```python
from build123d import *

# Parameters (mm, degrees)
BOSS_EXTRUDE1_DEPTH          = 40
SKETCH2_W                    = 3.5
SKETCH2_H                    = 40
BOSS_EXTRUDE2_DEPTH          = 5
SKETCH4_R                    = 2
CUT_EXTRUDE1_DEPTH           = 7
SKETCH5_R                    = 3.5
CUT_EXTRUDE2_DEPTH           = 3
CUT_EXTRUDE2_DRAFT           = -27
CUT_EXTRUDE2_PROFILE_2_DEPTH = 3
CUT_EXTRUDE2_PROFILE_2_DRAFT = -27
BOSS_EXTRUDE3_DEPTH          = 3
SKETCH9_W                    = 13
SKETCH9_H                    = 40
CUT_EXTRUDE4_DEPTH           = 4.702585656
SKETCH10_W                   = 15
SKETCH10_H                   = 40
BOSS_EXTRUDE4_DEPTH          = 2.5
SKETCH11_W                   = 1.5
SKETCH11_H                   = 2.202585656
BOSS_EXTRUDE7_DEPTH          = 40
BOSS_EXTRUDE8_DEPTH          = 0.625841469
SKETCH13_R                   = 2
CUT_EXTRUDE5_DEPTH           = 10
SKETCH14_W                   = 2.5
SKETCH14_H                   = 40
BOSS_EXTRUDE9_DEPTH          = 0.5
SKETCH15_W                   = 2.5
SKETCH15_H                   = 40
BOSS_EXTRUDE10_DEPTH         = 0.5
BOSS_EXTRUDE11_DEPTH         = 40
BOSS_EXTRUDE12_DEPTH         = 1.13137085
SKETCH18_R                   = 2
CUT_EXTRUDE6_DEPTH           = 10
SKETCH19_R                   = 3
CUT_EXTRUDE7_DEPTH           = 3
CUT_EXTRUDE7_DRAFT           = -19
CUT_EXTRUDE7_PROFILE_2_DEPTH = 3
CUT_EXTRUDE7_PROFILE_2_DRAFT = -19
SKETCH20_W                   = 5
SKETCH20_H                   = 40
BOSS_EXTRUDE13_DEPTH         = 0.5
SKETCH21_W                   = 5
SKETCH21_H                   = 40
BOSS_EXTRUDE14_DEPTH         = 0.5


with BuildPart() as part:
    # Sketch1 → Boss-Extrude1 (new body)
    with BuildSketch(Plane(origin=(0, 0, 0), x_dir=(1, 0, 0), z_dir=(0, 1, 0))):
        Polygon((-4.247892457, 4.702585656), (8.752107543, 4.702585656), (8.752107543, 1.702585656), (7.049521887, 0), (-2.545306801, 0), (-4.247892457, 1.702585656), align=None)
    extrude(amount=BOSS_EXTRUDE1_DEPTH)

    # Sketch2 → Boss-Extrude2 (add)
    with BuildSketch(Plane.XY):
        with Locations((4.002107543, 20)):
            Rectangle(SKETCH2_W, SKETCH2_H)
        with Locations((0.502107543, 20)):
            Rectangle(SKETCH2_W, SKETCH2_H)
    extrude(amount=BOSS_EXTRUDE2_DEPTH)

    # Sketch4 → Cut-Extrude1 (cut)
    with BuildSketch(Plane.XY.offset(5)):
        with Locations((2.252107543, 30)):
            Circle(SKETCH4_R)
        with Locations((2.252107543, 10)):
            Circle(SKETCH4_R)
    extrude(amount=-CUT_EXTRUDE1_DEPTH, mode=Mode.SUBTRACT)


with BuildPart() as cut_extrude2_tool:
    # Sketch5 → Cut-Extrude2 (with draft: the straight prism first)
    with BuildSketch(Plane(origin=(0, 0, -4.702585656), x_dir=(-1, 0, 0), z_dir=(0, 0, -1))):
        with Locations((-2.252107543, 30)):
            Circle(SKETCH5_R)
    extrude(amount=-CUT_EXTRUDE2_DEPTH)
    # Cut-Extrude2: the draft: its side faces are tilted about the plane it starts from
    cut_extrude2_sides = [cut_extrude2_tool.faces().sort_by_distance(p)[0] for p in [
        (5.752107543, 30, -3.202585656),
    ]]
    draft(cut_extrude2_sides, Plane(origin=(0, 0, -4.702585656), x_dir=(-1, 0, 0), z_dir=(0, 0, -1)), CUT_EXTRUDE2_DRAFT)


with BuildPart() as part_1:
    add(part.part)

    # Cut-Extrude2: cut by cut_extrude2_tool
    add(cut_extrude2_tool.part, mode=Mode.SUBTRACT)


with BuildPart() as cut_extrude2_profile_2_tool:
    # Sketch5 → Cut-Extrude2 profile 2 (with draft: the straight prism first)
    with BuildSketch(Plane(origin=(0, 0, -4.702585656), x_dir=(-1, 0, 0), z_dir=(0, 0, -1))):
        with Locations((-2.252107543, 10)):
            Circle(SKETCH5_R)
    extrude(amount=-CUT_EXTRUDE2_PROFILE_2_DEPTH)
    # Cut-Extrude2 profile 2: the draft: its side faces are tilted about the plane it starts from
    cut_extrude2_profile_2_sides = [cut_extrude2_profile_2_tool.faces().sort_by_distance(p)[0] for p in [
        (5.752107543, 10, -3.202585656),
    ]]
    draft(cut_extrude2_profile_2_sides, Plane(origin=(0, 0, -4.702585656), x_dir=(-1, 0, 0), z_dir=(0, 0, -1)), CUT_EXTRUDE2_PROFILE_2_DRAFT)


with BuildPart() as part_2:
    add(part_1.part)

    # Cut-Extrude2 profile 2: cut by cut_extrude2_profile_2_tool
    add(cut_extrude2_profile_2_tool.part, mode=Mode.SUBTRACT)

    # Sketch7 → Boss-Extrude3 (add)
    with BuildSketch(Plane(origin=(0, 0, -4.702585656), x_dir=(-1, 0, 0), z_dir=(0, 0, -1))):
        Polygon((1.247892457, 46.5), (-5.752107543, 46.5), (-5.752107543, 40), (-4.252107543, 40), (-4.252107543, 45), (-0.252107543, 45), (-0.252107543, 43.275204256), (-0.252107543, 40), (1.247892457, 40), align=None)
        Polygon((-4.252107543, 0), (-5.752107543, 0), (-5.752107543, -6.5), (1.247892457, -6.5), (1.247892457, 0), (-0.252107543, 0), (-0.252107543, -5), (-4.252107543, -5), align=None)
    extrude(amount=-BOSS_EXTRUDE3_DEPTH)

    # Sketch9 → Cut-Extrude4 (cut)
    with BuildSketch(Plane(origin=(0, 0, -4.702585656), x_dir=(-1, 0, 0), z_dir=(0, 0, -1))):
        with Locations((-2.252107543, 20)):
            Rectangle(SKETCH9_W, SKETCH9_H)
    extrude(amount=-CUT_EXTRUDE4_DEPTH, mode=Mode.SUBTRACT)


with BuildPart() as cut_extrude4_piece_1:
    # of the separate pieces the step leaves, piece 1, a body of its own (cut_extrude4_pieces)
    add(part_2.part.solids().sort_by_distance((-1.247892457, 0, 0))[0])



with BuildPart() as cut_extrude4_piece_2:
    # of the separate pieces the step leaves, piece 2, a body of its own (cut_extrude4_pieces)
    add(part_2.part.solids().sort_by_distance((0.252107543, 40, -4.702585656))[0])


with BuildPart() as cut_extrude4_piece_3:
    # of the separate pieces the step leaves, piece 3, a body of its own (cut_extrude4_pieces)
    add(part_2.part.solids().sort_by_distance((-1.247892457, -6.5, -4.702585656))[0])


with BuildPart() as cut_extrude4_piece_1_1:
    add(cut_extrude4_piece_1.part)

    add(cut_extrude4_piece_2.part)  # Boss-Extrude4 merges Cut-Extrude4 piece 2

    add(cut_extrude4_piece_3.part)  # Boss-Extrude4 merges Cut-Extrude4 piece 3
    # Sketch10 → Boss-Extrude4 (add)
    with BuildSketch(Plane(origin=(0, 0, 0), x_dir=(-1, 0, 0), z_dir=(0, 0, -1))):
        with Locations((-2.252107543, 20)):
            Rectangle(SKETCH10_W, SKETCH10_H)
    extrude(amount=BOSS_EXTRUDE4_DEPTH)

    # Sketch11 → Boss-Extrude7 (add)
    with BuildSketch(Plane(origin=(0, 0, 0), x_dir=(1, 0, 0), z_dir=(0, 1, 0))):
        with Locations((5.002107543, 3.601292828)):
            Rectangle(SKETCH11_W, SKETCH11_H)
        Polygon((-2.419465332, 5.328427125), (-5.247892457, 2.5), (4.252107543, 2.5), (4.252107543, 4.702585656), (5.752107543, 4.702585656), (5.752107543, 2.5), (9.752107543, 2.5), (6.923680418, 5.328427125), align=None)
    extrude(amount=BOSS_EXTRUDE7_DEPTH)

    # Sketch12 → Boss-Extrude8 (add)
    with BuildSketch(Plane(origin=(0, 0, -4.702585656), x_dir=(-1, 0, 0), z_dir=(0, 0, -1))):
        Polygon((-5.752107543, 0), (-5.752107543, -6.5), (1.247892457, -6.5), (1.247892457, 0), (-0.252107543, 0), (-0.252107543, -5), (-4.252107543, -5), (-4.252107543, 0), align=None)
        Polygon((1.247892457, 46.5), (-5.752107543, 46.5), (-5.752107543, 40), (-4.252107543, 40), (-4.252107543, 45), (-0.252107543, 45), (-0.252107543, 40), (1.247892457, 40), align=None)
    extrude(amount=BOSS_EXTRUDE8_DEPTH)

    # Sketch13 → Cut-Extrude5 (cut)
    with BuildSketch(Plane.XY):
        with Locations((2.252107543, 30)):
            Circle(SKETCH13_R)
        with Locations((2.252107543, 10)):
            Circle(SKETCH13_R)
    extrude(amount=-CUT_EXTRUDE5_DEPTH, mode=Mode.SUBTRACT)

    # Sketch14 → Boss-Extrude9 (add)
    with BuildSketch(Plane(origin=(9.752107543, 0, 0), x_dir=(0, 0, -1), z_dir=(1, 0, 0))):
        with Locations((1.25, 20)):
            Rectangle(SKETCH14_W, SKETCH14_H)
    extrude(amount=BOSS_EXTRUDE9_DEPTH)

    # Sketch15 → Boss-Extrude10 (add)
    with BuildSketch(Plane.ZY.offset(5.247892457)):
        with Locations((-1.25, 20)):
            Rectangle(SKETCH15_W, SKETCH15_H)
    extrude(amount=BOSS_EXTRUDE10_DEPTH)

    # Sketch16 → Boss-Extrude11 (add)
    with BuildSketch(Plane.XZ):
        Polygon((-2.419465332, -5.328427125), (-5.247892457, -2.5), (-5.747892457, -2.5), (-5.747892457, -3.13137085), (-2.419465332, -6.459797975), (6.923680418, -6.459797975), (10.252107543, -3.13137085), (10.252107543, -2.5), (9.752107543, -2.5), (6.923680418, -5.328427125), (0.656985658, -5.328427125), align=None)
    extrude(amount=-BOSS_EXTRUDE11_DEPTH)

    # Sketch17 → Boss-Extrude12 (add)
    with BuildSketch(Plane(origin=(0, 0, -5.328427125), x_dir=(-1, 0, 0), z_dir=(0, 0, -1))):
        Polygon((-5.752107543, 0), (-5.752107543, -6.5), (1.247892457, -6.5), (1.247892457, 0), (0, 0), (0, -5), (-0.252107543, -5), (-4.252107543, -5), (-4.252107543, 0), align=None)
        Polygon((1.247892457, 46.5), (-5.752107543, 46.5), (-5.752107543, 40), (-4.252107543, 40), (-4.252107543, 44.953142187), (-0.252107543, 44.953142187), (-0.252107543, 40), (1.247892457, 40), align=None)
    extrude(amount=BOSS_EXTRUDE12_DEPTH)

    # Sketch18 → Cut-Extrude6 (cut)
    with BuildSketch(Plane.XY.offset(-5.328427125)):
        with Locations((2.252107543, 30)):
            Circle(SKETCH18_R)
        with Locations((2.252107543, 10)):
            Circle(SKETCH18_R)
    extrude(amount=-CUT_EXTRUDE6_DEPTH, mode=Mode.SUBTRACT)


with BuildPart() as cut_extrude7_tool:
    # Sketch19 → Cut-Extrude7 (with draft: the straight prism first)
    with BuildSketch(Plane(origin=(0, 0, -6.459797975), x_dir=(-1, 0, 0), z_dir=(0, 0, -1))):
        with Locations((-2.252107543, 30)):
            Circle(SKETCH19_R)
    extrude(amount=-CUT_EXTRUDE7_DEPTH)
    # Cut-Extrude7: the draft: its side faces are tilted about the plane it starts from
    cut_extrude7_sides = [cut_extrude7_tool.faces().sort_by_distance(p)[0] for p in [
        (5.252107543, 30, -4.959797975),
    ]]
    draft(cut_extrude7_sides, Plane(origin=(0, 0, -6.459797975), x_dir=(-1, 0, 0), z_dir=(0, 0, -1)), CUT_EXTRUDE7_DRAFT)


with BuildPart() as cut_extrude4_piece_1_2:
    add(cut_extrude4_piece_1_1.part)

    # Cut-Extrude7: cut by cut_extrude7_tool
    add(cut_extrude7_tool.part, mode=Mode.SUBTRACT)


with BuildPart() as cut_extrude7_profile_2_tool:
    # Sketch19 → Cut-Extrude7 profile 2 (with draft: the straight prism first)
    with BuildSketch(Plane(origin=(0, 0, -6.459797975), x_dir=(-1, 0, 0), z_dir=(0, 0, -1))):
        with Locations((-2.252107543, 10)):
            Circle(SKETCH19_R)
    extrude(amount=-CUT_EXTRUDE7_PROFILE_2_DEPTH)
    # Cut-Extrude7 profile 2: the draft: its side faces are tilted about the plane it starts from
    cut_extrude7_profile_2_sides = [cut_extrude7_profile_2_tool.faces().sort_by_distance(p)[0] for p in [
        (5.252107543, 10, -4.959797975),
    ]]
    draft(cut_extrude7_profile_2_sides, Plane(origin=(0, 0, -6.459797975), x_dir=(-1, 0, 0), z_dir=(0, 0, -1)), CUT_EXTRUDE7_PROFILE_2_DRAFT)


with BuildPart() as cut_extrude4_piece_1_3:
    add(cut_extrude4_piece_1_2.part)

    # Cut-Extrude7 profile 2: cut by cut_extrude7_profile_2_tool
    add(cut_extrude7_profile_2_tool.part, mode=Mode.SUBTRACT)

    # Sketch20 → Boss-Extrude13 (add)
    with BuildSketch(Plane.ZY.offset(1.247892457)):
        with Locations((2.5, 20)):
            Rectangle(SKETCH20_W, SKETCH20_H)
    extrude(amount=BOSS_EXTRUDE13_DEPTH)

    # Sketch21 → Boss-Extrude14 (add)
    with BuildSketch(Plane(origin=(5.752107543, 0, 0), x_dir=(0, 0, -1), z_dir=(1, 0, 0))):
        with Locations((-2.5, 20)):
            Rectangle(SKETCH21_W, SKETCH21_H)
    extrude(amount=BOSS_EXTRUDE14_DEPTH)


solid = cut_extrude4_piece_1_3.part
```
Can you work these out from the model? Positions are in its coordinate system, mm. A direction names the side the tool comes from. Round coordinates to 2 decimals unless told otherwise and drop trailing zeros. Loops run counter-clockwise (first coordinate to the right, second up) from the corner with the lowest first, then second, coordinate; pieces in that order, holes last. Notation, with made-up numbers: M -39,89 L 19,89 A14 ccw 19,102 Z; hole C 76,50 d6. An arc over 180 degrees is marked long. Write item = value, one per line. Start each with the question number.
(1) Suppose I cut it at B-B on z = 2.25. Write out the boundary of the cut face in (x, y).
(2) I'm going to push flat-ended pins straight in: P1, Ø2.5, axis at y = 44.5, z = -5, coming from the +X side; P2, Ø2.5, axis at y = 10, z = 1.5, coming from the -X side; P3, Ø2.5, axis at y = -3.5, z = -4, coming from the -X side. Where does each tip first touch, or does it pass through?
(3) Which directions (+Z, -Z, +X, -X, +Y, -Y) give clear straight access to the entire face, cutting with the end or side of a thin tool? Please do faces 4 (the face through (8, 20, 0)), 5 (the face through (2.3, 45.5, -1.703)), 6 (the face through (2.3, -5.4, -1.703)), 7 (the face through (-1.248, 43, -4)), 8 (the face through (-4, 20, 0)).
(4) Suppose I cut it at C-C on y = 3. Write out the boundary of the cut face in (x, z).
(5) If we mould it in two halves opening along X, with no side actions, what happens to faces 1 (the face through (5.752, 43, -4)), 2 (the face through (2, 40, -1)), 3 (the face through (-1.248, -3, -4))? For each: released by +X, released by -X, zero draft, split by the parting line, or undercut.
(6) Suppose I cut it at A-A on y = 10. Write out the boundary of the cut face in (x, z), plus the area to 3 significant figures.
(7) I need wall thicknesses on line 1 along X through (y, z) = (30, 1); line 2 along X through (y, z) = (44, -3.75); line 3 along Y through (x, z) = (2.5, -2). Which ranges of each line are inside material? Lowest first, please.
Answer block:
q1.outline = M -1.75,0 L 6.25,0 L 6.25,40 L -1.75,40 Z; hole C 2.25,10 d4; hole C 2.25,30 d4
q2.P1 = 5.75
q2.P2 = -1.75
q2.P3 = -1.25
q3.face_4 = +Z, +X, +Y, -Y
q3.face_5 = +Z, +X, -X, +Y
q3.face_6 = +Z, +X, -X, -Y
q3.face_7 = +Z, -Z, -X, +Y
q3.face_8 = +Z, -X, +Y, -Y
q4.outline = M -5.75,-3.13 L -2.42,-6.46 L 6.92,-6.46 L 10.25,-3.13 L 10.25,0 L 6.25,0 L 6.25,5 L -1.75,5 L -1.75,0 L -5.75,0 Z
q5.face_1 = released by +X
q5.face_2 = undercut
q5.face_3 = released by -X
q6.outline = M -5.75,-3.13 L -2.42,-6.46 L -0.75,-6.46 L 0.25,-3.56 L 0.25,5 L -1.75,5 L -1.75,0 L -5.75,0 Z; M 4.25,-3.56 L 5.25,-6.46 L 6.92,-6.46 L 10.25,-3.13 L 10.25,0 L 6.25,0 L 6.25,5 L 4.25,5 Z
q6.area = 83.5 mm²
q7.line_1 = -1.75 to 0.25, 4.25 to 6.25
q7.line_2 = -1.25 to 0.25, 4.25 to 5.75
q7.line_3 = -6.5 to -5, 0 to 8.02, 11.98 to 28.02, 31.98 to 40, 45 to 46.5
